```python
from build123d import *

# Parameters (mm, degrees)
SKETCH1_R           = 2.3
BOSS_EXTRUDE1_DEPTH = 984.25


with BuildPart() as part:
    # Sketch1 → Boss-Extrude1 (new body)
    with BuildSketch(Plane.XY):
        with BuildLine():
            Line((14.58, -20), (18.5, -20))
            ThreePointArc((18.5, -20), (19.560660172, -19.560660172), (20, -18.5))
            Line((20, -18.5), (20, -14.58))
            Line((20, -14.58), (18.815, -13.395))
            Line((18.815, -13.395), (18.2, -13.395))
            Line((18.2, -13.395), (18.2, -15.5))
            Line((18.2, -15.5), (16.560660172, -15.5))
            Line((16.560660172, -15.5), (13.9, -12.839339828))
            Line((13.9, -12.839339828), (13.9, -10.21))
            Line((13.9, -10.21), (13.69, -10))
            Line((13.69, -10), (13.9, -9.79))
            Line((13.9, -9.79), (13.9, -7.160660172))
            Line((13.9, -7.160660172), (16.560660172, -4.5))
            Line((16.560660172, -4.5), (18.2, -4.5))
            Line((18.2, -4.5), (18.2, -6.605))
            Line((18.2, -6.605), (18.815, -6.605))
            Line((18.815, -6.605), (20, -5.42))
            Line((20, -5.42), (20, 5.42))
            Line((20, 5.42), (18.815, 6.605))
            Line((18.815, 6.605), (18.2, 6.605))
            Line((18.2, 6.605), (18.2, 4.5))
            Line((18.2, 4.5), (16.560660172, 4.5))
            Line((16.560660172, 4.5), (13.9, 7.160660172))
            Line((13.9, 7.160660172), (13.9, 9.79))
            Line((13.9, 9.79), (13.69, 10))
            Line((13.69, 10), (13.9, 10.21))
            Line((13.9, 10.21), (13.9, 12.839339828))
            Line((13.9, 12.839339828), (16.560660172, 15.5))
            Line((16.560660172, 15.5), (18.2, 15.5))
            Line((18.2, 15.5), (18.2, 13.395))
            Line((18.2, 13.395), (18.815, 13.395))
            Line((18.815, 13.395), (20, 14.58))
            Line((20, 14.58), (20, 18.5))
            ThreePointArc((20, 18.5), (19.560660172, 19.560660172), (18.5, 20))
            Line((18.5, 20), (14.58, 20))
            Line((14.58, 20), (13.395, 18.815))
            Line((13.395, 18.815), (13.395, 18.2))
            Line((13.395, 18.2), (15.5, 18.2))
            Line((15.5, 18.2), (15.5, 16.560660172))
            Line((15.5, 16.560660172), (12.839339828, 13.9))
            Line((12.839339828, 13.9), (10.21, 13.9))
            Line((10.21, 13.9), (10, 13.69))
            Line((10, 13.69), (9.79, 13.9))
            Line((9.79, 13.9), (7.160660172, 13.9))
            Line((7.160660172, 13.9), (4.5, 16.560660172))
            Line((4.5, 16.560660172), (4.5, 18.2))
            Line((4.5, 18.2), (6.605, 18.2))
            Line((6.605, 18.2), (6.605, 18.815))
            Line((6.605, 18.815), (5.42, 20))
            Line((5.42, 20), (-5.42, 20))
            Line((-5.42, 20), (-6.605, 18.815))
            Line((-6.605, 18.815), (-6.605, 18.2))
            Line((-6.605, 18.2), (-4.5, 18.2))
            Line((-4.5, 18.2), (-4.5, 16.560660172))
            Line((-4.5, 16.560660172), (-7.160660172, 13.9))
            Line((-7.160660172, 13.9), (-9.79, 13.9))
            Line((-9.79, 13.9), (-10, 13.69))
            Line((-10, 13.69), (-10.21, 13.9))
            Line((-10.21, 13.9), (-12.839339828, 13.9))
            Line((-12.839339828, 13.9), (-15.5, 16.560660172))
            Line((-15.5, 16.560660172), (-15.5, 18.2))
            Line((-15.5, 18.2), (-13.395, 18.2))
            Line((-13.395, 18.2), (-13.395, 18.815))
            Line((-13.395, 18.815), (-14.58, 20))
            Line((-14.58, 20), (-18.5, 20))
            ThreePointArc((-18.5, 20), (-19.560660172, 19.560660172), (-20, 18.5))
            Line((-20, 18.5), (-20, 14.58))
            Line((-20, 14.58), (-18.815, 13.395))
            Line((-18.815, 13.395), (-18.2, 13.395))
            Line((-18.2, 13.395), (-18.2, 15.5))
            Line((-18.2, 15.5), (-16.560660172, 15.5))
            Line((-16.560660172, 15.5), (-13.9, 12.839339828))
            Line((-13.9, 12.839339828), (-13.9, 10.21))
            Line((-13.9, 10.21), (-13.69, 10))
            Line((-13.69, 10), (-13.9, 9.79))
            Line((-13.9, 9.79), (-13.9, 7.160660172))
            Line((-13.9, 7.160660172), (-16.560660172, 4.5))
            Line((-16.560660172, 4.5), (-18.2, 4.5))
            Line((-18.2, 4.5), (-18.2, 6.605))
            Line((-18.2, 6.605), (-18.815, 6.605))
            Line((-18.815, 6.605), (-20, 5.42))
            Line((-20, 5.42), (-20, -5.42))
            Line((-20, -5.42), (-18.815, -6.605))
            Line((-18.815, -6.605), (-18.2, -6.605))
            Line((-18.2, -6.605), (-18.2, -4.5))
            Line((-18.2, -4.5), (-16.560660172, -4.5))
            Line((-16.560660172, -4.5), (-13.9, -7.160660172))
            Line((-13.9, -7.160660172), (-13.9, -9.79))
            Line((-13.9, -9.79), (-13.69, -10))
            Line((-13.69, -10), (-13.9, -10.21))
            Line((-13.9, -10.21), (-13.9, -12.839339828))
            Line((-13.9, -12.839339828), (-16.560660172, -15.5))
            Line((-16.560660172, -15.5), (-18.2, -15.5))
            Line((-18.2, -15.5), (-18.2, -13.395))
            Line((-18.2, -13.395), (-18.815, -13.395))
            Line((-18.815, -13.395), (-20, -14.58))
            Line((-20, -14.58), (-20, -18.5))
            ThreePointArc((-20, -18.5), (-19.560660172, -19.560660172), (-18.5, -20))
            Line((-18.5, -20), (-14.58, -20))
            Line((-14.58, -20), (-13.395, -18.815))
            Line((-13.395, -18.815), (-13.395, -18.2))
            Line((-13.395, -18.2), (-15.5, -18.2))
            Line((-15.5, -18.2), (-15.5, -16.560660172))
            Line((-15.5, -16.560660172), (-12.839339828, -13.9))
            Line((-12.839339828, -13.9), (-10.21, -13.9))
            Line((-10.21, -13.9), (-10, -13.69))
            Line((-10, -13.69), (-9.79, -13.9))
            Line((-9.79, -13.9), (-7.160660172, -13.9))
            Line((-7.160660172, -13.9), (-4.5, -16.560660172))
            Line((-4.5, -16.560660172), (-4.5, -18.2))
            Line((-4.5, -18.2), (-6.605, -18.2))
            Line((-6.605, -18.2), (-6.605, -18.815))
            Line((-6.605, -18.815), (-5.42, -20))
            Line((-5.42, -20), (5.42, -20))
            Line((5.42, -20), (6.605, -18.815))
            Line((6.605, -18.815), (6.605, -18.2))
            Line((6.605, -18.2), (4.5, -18.2))
            Line((4.5, -18.2), (4.5, -16.560660172))
            Line((4.5, -16.560660172), (7.160660172, -13.9))
            Line((7.160660172, -13.9), (9.79, -13.9))
            Line((9.79, -13.9), (10, -13.69))
            Line((10, -13.69), (10.21, -13.9))
            Line((10.21, -13.9), (12.839339828, -13.9))
            Line((12.839339828, -13.9), (15.5, -16.560660172))
            Line((15.5, -16.560660172), (15.5, -18.2))
            Line((15.5, -18.2), (13.395, -18.2))
            Line((13.395, -18.2), (13.395, -18.815))
            Line((13.395, -18.815), (14.58, -20))
        make_face()
        with Locations((-10, -10)):
            Circle(SKETCH1_R, mode=Mode.SUBTRACT)
        with Locations((10, -10)):
            Circle(SKETCH1_R, mode=Mode.SUBTRACT)
        Polygon((-16.239339828, -2.7), (-18.2, -2.7), (-18.2, 2.7), (-16.239339828, 2.7), (-12.839339828, 6.1), (-7.160660172, 6.1), (-6.1, 7.160660172), (-6.1, 12.839339828), (-2.7, 16.239339828), (-2.7, 18.2), (2.7, 18.2), (2.7, 16.239339828), (6.1, 12.839339828), (6.1, 7.160660172), (7.160660172, 6.1), (12.839339828, 6.1), (16.239339828, 2.7), (18.2, 2.7), (18.2, -2.7), (16.239339828, -2.7), (12.839339828, -6.1), (7.160660172, -6.1), (6.1, -7.160660172), (6.1, -12.839339828), (2.7, -16.239339828), (2.7, -18.2), (-2.7, -18.2), (-2.7, -16.239339828), (-6.1, -12.839339828), (-6.1, -7.160660172), (-7.160660172, -6.1), (-12.839339828, -6.1), align=None, mode=Mode.SUBTRACT)
        with Locations((-10, 10)):
            Circle(SKETCH1_R, mode=Mode.SUBTRACT)
        with Locations((10, 10)):
            Circle(SKETCH1_R, mode=Mode.SUBTRACT)
    extrude(amount=BOSS_EXTRUDE1_DEPTH)


solid = part.part
```
Work out the finished part from the listing and answer in its coordinate system (mm). Round coordinates to 2 decimals unless told otherwise and drop trailing zeros. Return JSON: item names as keys, results as strings. Group by question number.
Q1. Find the intervals of material crossed by L1, parallel to X at y = -6.5, z = 282; L2, parallel to X at y = -13.5, z = 278.5; L3, parallel to Y at x = 10, z = 654, in increasing order.
Q2. The part is cut by section A-A on z = 355.5. Count the separate pieces of the cut face and the enclosed holes in it, then the cut area to 3 significant figures.
Q3. Each of these flat-tipped pins is pushed along its axis until it touches: pin 1 Ø0.6 at (x, z) = (-6, 506) entering from -Y; pin 2 Ø0.8 at (y, z) = (-11, 485.5) entering from -X; pin 3 Ø8 at (x, y) = (-5.5, 1.5) entering from +Z; pin 4 Ø3 at (y, z) = (-10.5, 854) entering from +X. Where does it stop, or does it pass through?
Solved:
{
 "1": {"L1": "-18.92 to -18.2, -14.56 to -6.76, 6.76 to 14.56, 18.2 to 18.92", "L2": "-18.92 to -18.2, -14.56 to -5.44, 5.44 to 14.56, 18.2 to 18.92", "L3": "-13.69 to -12.3, -7.7 to -6.1, 6.1 to 7.7, 12.3 to 13.69"},
 "2": {"separate pieces": "1", "enclosed holes": "5", "area": "458 mm²"},
 "3": {"pin 1": "y = -19.72", "pin 2": "x = -13.9", "pin 3": "through", "pin 4": "x = 13.9"}
}
